Model file for the job. Use its own axes, mm. A direction names the side the tool comes from. Round coordinates to 2 decimals unless told otherwise and drop trailing zeros. Order: outer loops, then holes, each group sorted by start corner. A loop starts at its lowest first (then second) coordinate and runs counter-clockwise, first axis right, second up. Notation, with made-up numbers: (-27, 11) -> (9, 11) arc R20 cw to (9, 27) -> close; hole circle Ø2 at (-23, -9.5). An arc over 180 degrees is marked (long way). Answer as CSV lines item,"result".
```python
from build123d import *
from OCP.BRepFilletAPI import BRepFilletAPI_MakeChamfer

# Parameters (mm, degrees)
SKETCH1_W            = 69.35
SKETCH1_H            = 113.5
BOSS_EXTRUDE5_DEPTH  = 2
SKETCH2_R            = 2.35
CUT_EXTRUDE3_DEPTH   = 2.5
FACE_CHAMFER_SIZE    = 1.5
FACE_CHAMFER_SIZE2   = 1.258649447
SKETCH4_W            = 60.238416088
SKETCH4_H            = 90.514495008
CUT_EXTRUDE6_DEPTH   = 1.5
SKETCH5_W            = 20.93325514
SKETCH5_H            = 17.0989254
SKETCH5_W_2          = 13.4
SKETCH5_H_2          = 10.2
BOSS_EXTRUDE7_DEPTH  = 4.5
SKETCH6_W            = 13.4
SKETCH6_H            = 10.2
CUT_EXTRUDE7_DEPTH   = 4.1
SKETCH7_W            = 20.93325514
SKETCH7_H            = 17.0989254
BOSS_EXTRUDE8_DEPTH  = 0.5
SKETCH8_W            = 2.621357244
SKETCH8_H            = 10.2
CUT_EXTRUDE8_DEPTH   = 0.5
SKETCH10_W           = 1.18316995
SKETCH10_H           = 0.660821766
BOSS_EXTRUDE11_DEPTH = 1
FILLET1_R            = 0.9


with BuildPart() as part:
    # Sketch1 → Boss-Extrude5 (new body)
    with BuildSketch(Plane(origin=(0, 0, 0), x_dir=(1, 0, 0), z_dir=(0, 1, 0))):
        Rectangle(SKETCH1_W, SKETCH1_H)
    extrude(amount=BOSS_EXTRUDE5_DEPTH)

    # Sketch2 → Cut-Extrude3 (cut)
    with BuildSketch(Plane(origin=(0, 2, 0), x_dir=(1, 0, 0), z_dir=(0, 1, 0))):
        with Locations(Location((0, 48.943079059, 0), (0, 0, 270))):
            Circle(SKETCH2_R)
        with Locations(Location((0, -48.943079059, 0), (0, 0, 90))):
            Circle(SKETCH2_R)
    extrude(amount=-CUT_EXTRUDE3_DEPTH, mode=Mode.SUBTRACT)

    # face chamfer: one chamfer whose edges measure the first distance from different faces: ONE call of the kernel's chamfer builder (chamfer() names one face for all edges)
    face_chamfer_edges_1 = [part.edges().sort_by_distance(p)[0] for p in [
        (0, 2, -56.75),
        (-34.675, 2, 0),
        (0, 2, 56.75),
        (34.675, 2, 0),
    ]]
    face_chamfer_side_1 = [part.faces().sort_by_distance(p)[0] for p in [
        (0, 2, 0),
    ]]
    face_chamfer_edges_2 = [part.edges().sort_by_distance(p)[0] for p in [
        (0, 2, -51.293079059),
    ]]
    face_chamfer_side_2 = [part.faces().sort_by_distance(p)[0] for p in [
        (0, 1, -51.293079059),
    ]]
    face_chamfer_edges_3 = [part.edges().sort_by_distance(p)[0] for p in [
        (0, 2, 51.293079059),
    ]]
    face_chamfer_side_3 = [part.faces().sort_by_distance(p)[0] for p in [
        (0, 1, 51.293079059),
    ]]
    face_chamfer = BRepFilletAPI_MakeChamfer(part.part.solid().wrapped)
    for e in face_chamfer_edges_1:
        face_chamfer.Add(FACE_CHAMFER_SIZE, FACE_CHAMFER_SIZE2, e.wrapped, face_chamfer_side_1[0].wrapped)  # the first distance lies on this face
    for e in face_chamfer_edges_2:
        face_chamfer.Add(FACE_CHAMFER_SIZE, FACE_CHAMFER_SIZE2, e.wrapped, face_chamfer_side_2[0].wrapped)  # the first distance lies on this face
    for e in face_chamfer_edges_3:
        face_chamfer.Add(FACE_CHAMFER_SIZE, FACE_CHAMFER_SIZE2, e.wrapped, face_chamfer_side_3[0].wrapped)  # the first distance lies on this face
    add(Compound.cast(face_chamfer.Shape()), mode=Mode.REPLACE)

    # Sketch4 → Cut-Extrude6 (cut)
    with BuildSketch(Plane(origin=(0, 0, 0), x_dir=(-1, 0, 0), z_dir=(0, -1, 0))):
        Rectangle(SKETCH4_W, SKETCH4_H)
    extrude(amount=-CUT_EXTRUDE6_DEPTH, mode=Mode.SUBTRACT)

    # Sketch5 → Boss-Extrude7 (add)
    with BuildSketch(Plane(origin=(0, 2, 0), x_dir=(1, 0, 0), z_dir=(0, 1, 0))):
        Rectangle(SKETCH5_W, SKETCH5_H)
        Rectangle(SKETCH5_W_2, SKETCH5_H_2, mode=Mode.SUBTRACT)
    extrude(amount=-BOSS_EXTRUDE7_DEPTH)

    # Sketch6 → Cut-Extrude7 (cut)
    with BuildSketch(Plane(origin=(0, 2, 0), x_dir=(1, 0, 0), z_dir=(0, 1, 0))):
        Rectangle(SKETCH6_W, SKETCH6_H)
    extrude(amount=-CUT_EXTRUDE7_DEPTH, mode=Mode.SUBTRACT)

    # Sketch7 → Boss-Extrude8 (add)
    with BuildSketch(Plane.XZ.offset(2.5)):
        Rectangle(SKETCH7_W, SKETCH7_H)
    extrude(amount=BOSS_EXTRUDE8_DEPTH)

    # Sketch8 → Cut-Extrude8 (cut)
    with BuildSketch(Plane(origin=(0, -2.5, 0), x_dir=(1, 0, 0), z_dir=(0, 1, 0))):
        with Locations((-5.389321378, 0)):
            Rectangle(SKETCH8_W, SKETCH8_H)
    extrude(amount=-CUT_EXTRUDE8_DEPTH, mode=Mode.SUBTRACT)

    # Sketch10 → Boss-Extrude11 (add)
    with BuildSketch(Plane.ZY.offset(-6.7)):
        with Locations((-0.045919003, 0.630410883)):
            Rectangle(SKETCH10_W, SKETCH10_H)
    extrude(amount=BOSS_EXTRUDE11_DEPTH)

    # Fillet1
    # the kernel refuses this fillet: 0.9 mm, written as the material it takes off along each edge
    with BuildSketch(Plane(origin=(5.7, 0.960821766, 2.714758197), x_dir=(1, 0, 0), z_dir=(0, 0, -1))) as fillet1_piece_1:
        with BuildLine():
            CenterArc((0.86763689, 0.9), FILLET1_R, 195.411736224, 74.588263776)
            Line((0, 0.660821766), (-0.017352738, 0.656038202))
            ThreePointArc((-0.017352738, 0.656038202), (-0.018, 0.330410883), (-0.018, 0))
            Line((-0.018, 0), (0, -0.018))
            Line((0, -0.018), (0.86763689, -0.018))
            Line((0.86763689, -0.018), (0.86763689, 0))
        make_face()
    extrude(amount=5.521354399, mode=Mode.SUBTRACT)


solid = part.part
```
Q1. Saw through at B-B (y = -1.2). Write the cut outline in (x, z).
Checks:
outline,"(-10.47, -8.55) -> (10.47, -8.55) -> (10.47, 8.55) -> (-10.47, 8.55) -> close; hole (-6.7, -5.1) -> (6.7, -5.1) -> (6.7, 5.1) -> (-6.7, 5.1) -> close"
Q2. Wall check: L1, parallel to Z at x = -21.5, y = 0.05; L2, parallel to Z at x = 4, y = -1.3; L3, parallel to Y at x = 10.5, z = -40. Give the ranges that are in metal, low to high. Write a range as [from, to].
Checks:
L1,"[-56.75, -45.26], [45.26, 56.75]"
L2,"[-8.55, -5.1], [5.1, 8.55]"
L3,"[1.5, 2]"
Q3. Tool access for faces 1 (the flat face through (0, 0, -5.1)), 2 (the flat face through (10.467, -1, 0)), 3 (the flat face through (7, 2, -1)), 4 (the flat face through (-6.7, 0, 0)): list every direction of +Z, -Z, +X, -X, +Y, -Y with a clear straight run to the whole face (end or side of a thin tool).
Checks:
face 1,"+Y"
face 2,"-Y"
face 3,"+Z, -Z, +X, -X, +Y"
face 4,"+Y, -Y"
Q4. Saw through at C-C (x = 0). State how many separate pieces and enclosed holes the cut face has, plus the area to 3 significant figures.
Checks:
separate pieces,"3"
enclosed holes,"0"
area,"97.8 mm²"
Q5. Saw through at D-D (z = -36). Write the cut outline in (x, y) (3 decimals), plus the area to 3 significant figures.
Checks:
outline,"(-34.675, 0) -> (-30.119, 0) -> (-30.119, 1.5) -> (30.119, 1.5) -> (30.119, 0) -> (34.675, 0) -> (34.675, 0.741) -> (33.175, 2) -> (-33.175, 2) -> (-34.675, 0.741) -> close"
area,"46.5 mm²"
Q6. Mould opens along Z. For faces 5 (the flat face through (0, -3, 0)), 6 (the cylindrical face through (1.43, 0.25, 50.81)) say: +Z half, -Z half, draft (parallel to the pull), parting line (faces both ways), or undercut.
Checks:
face 5,"draft"
face 6,"undercut"
Q7. Flat gauge pins, fed straight in: pin 1 (6 mm diameter, centred on x = -22.5, z = 34.5, fed in from -Y); pin 2 (5 mm diameter, centred on x = 3.5, z = -2, fed in from +Y); pin 3 (1.3 mm diameter, centred on x = 5, y = -1, fed in from +Z). Where does each tip first touch, or does it go through?
Checks:
pin 1,"y = 1.5"
pin 2,"y = -2.5"
pin 3,"z = 8.55"
Q8. Saw through at A-A (z = -4). Write the cut outline in (x, y) (3 decimals), plus the area to 3 significant figures.
Checks:
outline,"(-34.675, 0) -> (-30.119, 0) -> (-30.119, 1.5) -> (-10.467, 1.5) -> (-10.467, -3) -> (-6.7, -3) -> (-6.7, 2) -> (-33.175, 2) -> (-34.675, 0.741) -> close; (-4.079, -3) -> (10.467, -3) -> (10.467, 1.5) -> (30.119, 1.5) -> (30.119, 0) -> (34.675, 0) -> (34.675, 0.741) -> (33.175, 2) -> (6.7, 2) -> (6.7, -2.5) -> (-4.079, -2.5) -> close"
area,"79.0 mm²"
